Input: part model. Units: mm. Frame: model coordinates. Face numbers are marked on the shaded views. A direction names the side the tool comes from. Coordinates: 2 decimals unless noted, no trailing zeros. Order: outer loops, then holes, each group sorted by start corner. A loop starts at its lowest first (then second) coordinate and runs counter-clockwise, first axis right, second up. Notation, with made-up numbers: (65.5, 20) - (106.5, 20) arc R8 cw to (106.5, 33) - close; hole circle Ø5 at (57, -38.5). An arc over 180 degrees is marked (long way). Answer as CSV lines item,"result". Start each with the question number.
Item 1: Material intervals for line 1 along X through (y, z) = (37.5, 5.5); line 2 along Y through (x, z) = (1, 9.5); line 3 along Z through (x, y) = (-7, 48), sorted ascending.
Item 2: Section A-A (y = 69.5). Output: boundary loops of the cut face in (x, z), and give its area (3 significant figures).
Item 3: Section C-C (z = 12.75). Output: boundary loops of the cut face in (x, y).
Item 4: Access query for the marked faces 5, 6, 7, 8 and 9. Directions: +Z, -Z, +X, -X, +Y, -Y. A direction counts if a zero-diameter tool reaches every point of the face in a straight line with its end or side. Return the directions, or none.
Item 5: Section B-B (x = 11). Output: boundary loops of the cut face in (y, z), and give its area (3 significant figures).
Item 6: First-contact query: pin 1 (3 mm diameter, centred on y = 63, z = 19.5, fed in from +X); pin 2 (0.7 mm diameter, centred on x = 8.5, z = 21.5, fed in from +Y); pin 3 (12 mm diameter, centred on x = -1.5, z = 12.5, fed in from -Y); pin 4 (8 mm diameter, centred on x = 23.5, z = 13.5, fed in from -Y). Flat tips, straight axial feed; report the tip coordinate or a pass-through.
Item 7: Draft query along Y for the marked faces 1, 2, 3 and 4. Return one class per face: +Y half, -Y half, draft (parallel to the pull), parting line (faces both ways), or undercut.
Item 8: Section D-D (x = 22.6). Output: boundary loops of the cut face in (y, z).
from build123d import *

# Parameters (mm, degrees)
EXTRUDE_1_DEPTH      = 30
SKETCH_2_W           = 20.2
SKETCH_2_H           = 50
EXTRUDE_1_2_DEPTH    = 20
SKETCH_3_W           = 20.2
SKETCH_3_H           = 11
CUT_EXTRUDE_1_DEPTH  = 20
CUT_EXTRUDE_2_REACH  = 60.432
SKETCH_4_W           = 11
SKETCH_4_H           = 20
SKETCH_5_W           = 20.2
SKETCH_5_H           = 4.5
EXTRUDE_2_DEPTH      = 25
CUT_EXTRUDE_4_REACH  = 80.275
CUT_EXTRUDE_5_REACH  = 82.278
SKETCH_9_R           = 1.6
SKETCH_10_W          = 20.2
SKETCH_10_H          = 20
EXTRUDE_3_DEPTH      = 3
CUT_EXTRUDE_6_REACH  = 55.965
SKETCH_12_W          = 20.2
SKETCH_12_H          = 30
EXTRUDE_4_DEPTH      = 2
SKETCH_13_W          = 20.2
SKETCH_13_H          = 30
EXTRUDE_5_DEPTH      = 2
CUT_EXTRUDE_START    = -20.2
SKETCH_15_W          = 15.2
SKETCH_15_H          = 20
CUT_EXTRUDE_7_DEPTH  = 20.2
SKETCH_16_W          = 4.4
SKETCH_16_H          = 30
SKETCH_16_W_2        = 5.4
EXTRUDE_6_DEPTH      = 20
CUT_EXTRUDE_8_REACH  = 88.983
SKETCH_17_R          = 1.6
CHAMFER_1_SIZE       = 2.5
CUT_EXTRUDE_9_REACH  = 89.122
SKETCH_18_W          = 46.30929367
SKETCH_18_H          = 3
SKETCH_20_W          = 20.2
SKETCH_20_H          = 20
EXTRUDE_7_DEPTH      = 2.1
SKETCH_21_W          = 20.2
SKETCH_21_H          = 20
EXTRUDE_8_DEPTH      = 2.1
SKETCH_22_W          = 46.206629154
SKETCH_22_H          = 1
CUT_EXTRUDE_10_DEPTH = 30
SKETCH_23_W          = 42.922328926
SKETCH_23_H          = 4
CUT_EXTRUDE_11_DEPTH = 30
CUT_EXTRUDE_12_REACH = 85.656
SKETCH_24_W          = 4
SKETCH_24_H          = 48
SKETCH_25_W          = 15.2
SKETCH_25_H          = 20
CUT_EXTRUDE_13_DEPTH = 20.2
SKETCH_26_W          = 20.2
SKETCH_26_H          = 20
EXTRUDE_9_DEPTH      = 1
CHAMFER_2_SIZE       = 2
FILLET_1_R           = 1
CUT_EXTRUDE_14_DEPTH = 1


with BuildPart() as part:
    # Sketch 1 → Extrude 1 (new body)
    with BuildSketch(Plane(origin=(0, 0, 0), x_dir=(1, 0, 0), z_dir=(0, 1, 0))):
        Polygon((-7.6, 15), (-7.6, 0), (7.6, 0), (7.6, 15), (10.1, 15), (10.1, -2.5), (-10.1, -2.5), (-10.1, 15), align=None)
    extrude(amount=EXTRUDE_1_DEPTH)

    # Sketch 2 → Extrude 1 2 (add)
    with BuildSketch(Plane.XY.offset(2.5)):
        with Locations((0, 25)):
            Rectangle(SKETCH_2_W, SKETCH_2_H)
    extrude(amount=EXTRUDE_1_2_DEPTH)

    # Sketch 3 → Cut-Extrude 1 (cut)
    with BuildSketch(Plane(origin=(0, 50, 0), x_dir=(1, 0, 0), z_dir=(0, 1, 0))):
        with Locations((0, -12.5)):
            Rectangle(SKETCH_3_W, SKETCH_3_H)
    extrude(amount=-CUT_EXTRUDE_1_DEPTH, mode=Mode.SUBTRACT)

    # Sketch 4 → Cut-Extrude 2 (cut, up to next)
    with BuildSketch(Plane(origin=(10.1, 0, 0), x_dir=(0, 0, -1), z_dir=(1, 0, 0)), mode=Mode.PRIVATE) as cut_extrude_2_sk1:
        with Locations((-12.5, 15)):
            Rectangle(SKETCH_4_W, SKETCH_4_H)
    cut_extrude_2_tool1 = extrude(cut_extrude_2_sk1.sketch, amount=-CUT_EXTRUDE_2_REACH, mode=Mode.PRIVATE) & part.part
    add(cut_extrude_2_tool1.solids().sort_by_distance((10.1, 15, 12.5))[0], mode=Mode.SUBTRACT)

    # Sketch 5 → Extrude 2 (add)
    with BuildSketch(Plane(origin=(0, 50, 0), x_dir=(1, 0, 0), z_dir=(0, 1, 0))):
        with Locations((0, -4.75)):
            Rectangle(SKETCH_5_W, SKETCH_5_H)
        with Locations((0, -20.25)):
            Rectangle(SKETCH_5_W, SKETCH_5_H)
    extrude(amount=EXTRUDE_2_DEPTH)

    # Sketch 7 → Hole Wizard M3.5 _1 (revolve, cut)
    with BuildSketch(Plane(origin=(-5.1, 37.5, 2.5), x_dir=(0, 1, 0), z_dir=(1, 0, 0))):
        Polygon((0, 0), (0, 40.871247898), (1.45, 40), (1.45, 0), align=None)
    hole_wizard_m3_5_1 = revolve(axis=Axis((-5.1, 37.5, -3.85), (0, 0, 1)), mode=Mode.SUBTRACT)

    # Cut-Extrude 4: up to this face of the body (flat: up to its plane)
    cut_extrude_4_end = Plane(part.part.faces().sort_by_distance((0.022332689, 37.5, 22.5))[0])
    # Sketch 8 → Cut-Extrude 4 (cut, up to the picked face)
    with BuildSketch(Plane(origin=(0, 0, 2.5), x_dir=(-1, 0, 0), z_dir=(0, 0, -1)), mode=Mode.PRIVATE) as cut_extrude_4_sk1:
        with BuildLine():
            Line((3.5, 60.5), (3.5, 64.5))
            ThreePointArc((3.5, 64.5), (5.1, 66.1), (6.7, 64.5))
            Line((6.7, 64.5), (6.7, 60.5))
            ThreePointArc((6.7, 60.5), (5.1, 58.9), (3.5, 60.5))
        make_face()
    cut_extrude_4_tool1 = split(extrude(cut_extrude_4_sk1.sketch, amount=-CUT_EXTRUDE_4_REACH, mode=Mode.PRIVATE), bisect_by=cut_extrude_4_end, keep=Keep.BOTH, mode=Mode.PRIVATE)
    cut_extrude_4 = cut_extrude_4_tool1.solids().sort_by(Axis((-5.1, 62.5, 2.5), (0, 0, 1)))[0]
    add(cut_extrude_4, mode=Mode.SUBTRACT)

    # Sketch 9 → Cut-Extrude 5 (cut, up to next)
    with BuildSketch(Plane(origin=(-7.6, 0, 0), x_dir=(0, 0, -1), z_dir=(1, 0, 0)), mode=Mode.PRIVATE) as cut_extrude_5_sk1:
        with Locations((7.5, 25)):
            Circle(SKETCH_9_R)
    cut_extrude_5_tool1 = extrude(cut_extrude_5_sk1.sketch, amount=-CUT_EXTRUDE_5_REACH, mode=Mode.PRIVATE) & part.part
    # Sketch 9 → Cut-Extrude 5 (cut, up to next)
    with BuildSketch(Plane(origin=(-7.6, 0, 0), x_dir=(0, 0, -1), z_dir=(1, 0, 0)), mode=Mode.PRIVATE) as cut_extrude_5_sk2:
        with Locations((7.5, 5)):
            Circle(SKETCH_9_R)
    cut_extrude_5_tool2 = extrude(cut_extrude_5_sk2.sketch, amount=-CUT_EXTRUDE_5_REACH, mode=Mode.PRIVATE) & part.part
    cut_extrude_5_1 = cut_extrude_5_tool1.solids().sort_by_distance((-7.6, 25, -7.5))[0]
    add(cut_extrude_5_1, mode=Mode.SUBTRACT)
    cut_extrude_5_2 = cut_extrude_5_tool2.solids().sort_by_distance((-7.6, 5, -7.5))[0]
    add(cut_extrude_5_2, mode=Mode.SUBTRACT)
    cut_extrude_5 = cut_extrude_5_1 + cut_extrude_5_2  # Cut-Extrude 5 as one shape, for the pattern or mirror that repeats it

    # Mirror 1: Hole Wizard M3.5 _1, Cut-Extrude 4, Cut-Extrude 5 across plane
    add(hole_wizard_m3_5_1.mirror(Plane(origin=(0, 0, 0), x_dir=(0, 0, 1), z_dir=(1, 0, 0))), mode=Mode.SUBTRACT)
    add(cut_extrude_4.mirror(Plane(origin=(0, 0, 0), x_dir=(0, 0, 1), z_dir=(1, 0, 0))), mode=Mode.SUBTRACT)
    add(cut_extrude_5.mirror(Plane(origin=(0, 0, 0), x_dir=(0, 0, 1), z_dir=(1, 0, 0))), mode=Mode.SUBTRACT)

    # Sketch 10 → Extrude 3 (add)
    with BuildSketch(Plane(origin=(0, 75, 0), x_dir=(1, 0, 0), z_dir=(0, 1, 0))):
        with Locations((0, -12.5)):
            Rectangle(SKETCH_10_W, SKETCH_10_H)
    extrude(amount=EXTRUDE_3_DEPTH)

    # Sketch 11 → Cut-Extrude 6 (cut, up to next)
    with BuildSketch(Plane(origin=(0, 30, 0), x_dir=(1, 0, 0), z_dir=(0, 1, 0)), mode=Mode.PRIVATE) as cut_extrude_6_sk1:
        Polygon((10.1, -2.5), (10.1, 15), (7.6, 15), (7.6, 0), (-7.6, 0), (-7.6, 15), (-10.1, 15), (-10.1, -2.5), align=None)
    cut_extrude_6_tool1 = extrude(cut_extrude_6_sk1.sketch, amount=-CUT_EXTRUDE_6_REACH, mode=Mode.PRIVATE) & part.part
    add(cut_extrude_6_tool1.solids().sort_by_distance((9.832738, 30, -6.25))[0], mode=Mode.SUBTRACT)

    # Sketch 12 → Extrude 4 (add)
    with BuildSketch(Plane.XY.offset(22.5)):
        with Locations((0, 15)):
            Rectangle(SKETCH_12_W, SKETCH_12_H)
    extrude(amount=EXTRUDE_4_DEPTH)

    # Sketch 13 → Extrude 5 (add)
    with BuildSketch(Plane(origin=(0, 0, 2.5), x_dir=(-1, 0, 0), z_dir=(0, 0, -1))):
        with Locations((0, 15)):
            Rectangle(SKETCH_13_W, SKETCH_13_H)
    extrude(amount=EXTRUDE_5_DEPTH)

    # Sketch 15 → Cut-Extrude 7 (cut)
    with BuildSketch(Plane(origin=(10.1, 0, 0), x_dir=(0, 0, -1), z_dir=(1, 0, 0)).offset(CUT_EXTRUDE_START)):
        with Locations((-12.5, 15)):
            Rectangle(SKETCH_15_W, SKETCH_15_H)
    extrude(amount=CUT_EXTRUDE_7_DEPTH, mode=Mode.SUBTRACT)

    # Sketch 16 → Extrude 6 (add)
    with BuildSketch(Plane(origin=(10.1, 0, 0), x_dir=(0, 0, -1), z_dir=(1, 0, 0))):
        with Locations((-22.3, 15)):
            Rectangle(SKETCH_16_W, SKETCH_16_H)
        with Locations((-3.2, 15)):
            Rectangle(SKETCH_16_W_2, SKETCH_16_H)
    extrude(amount=EXTRUDE_6_DEPTH)

    # Cut-Extrude 8: up to this face of the body (flat: up to its plane)
    cut_extrude_8_end = Plane(part.part.faces().sort_by_distance((10, 15, 0.5))[0])
    # Sketch 17 → Cut-Extrude 8 (cut, up to the picked face)
    with BuildSketch(Plane.XY.offset(24.5), mode=Mode.PRIVATE) as cut_extrude_8_sk1:
        with Locations((22.6, 25)):
            Circle(SKETCH_17_R)
    cut_extrude_8_tool1 = split(extrude(cut_extrude_8_sk1.sketch, amount=-CUT_EXTRUDE_8_REACH, mode=Mode.PRIVATE), bisect_by=cut_extrude_8_end, keep=Keep.BOTH, mode=Mode.PRIVATE)
    # Sketch 17 → Cut-Extrude 8 (cut, up to the picked face)
    with BuildSketch(Plane.XY.offset(24.5), mode=Mode.PRIVATE) as cut_extrude_8_sk2:
        with Locations((22.6, 5)):
            Circle(SKETCH_17_R)
    cut_extrude_8_tool2 = split(extrude(cut_extrude_8_sk2.sketch, amount=-CUT_EXTRUDE_8_REACH, mode=Mode.PRIVATE), bisect_by=cut_extrude_8_end, keep=Keep.BOTH, mode=Mode.PRIVATE)
    add(cut_extrude_8_tool1.solids().sort_by(Axis((22.6, 25, 24.5), (0, 0, -1)))[0], mode=Mode.SUBTRACT)
    add(cut_extrude_8_tool2.solids().sort_by(Axis((22.6, 5, 24.5), (0, 0, -1)))[0], mode=Mode.SUBTRACT)

    # Chamfer 1
    chamfer_1_edges = [part.edges().sort_by_distance(p)[0] for p in [
        (30.1, 0, 22.3),
        (30.1, 0, 3.2),
        (30.1, 30, 3.2),
        (30.1, 30, 22.3),
    ]]
    chamfer(chamfer_1_edges, length=CHAMFER_1_SIZE)

    # Cut-Extrude 9: up to this face of the body (flat: up to its plane)
    cut_extrude_9_end = Plane(part.part.faces().sort_by_distance((0, 78, 12.5))[0])
    # Sketch 18 → Cut-Extrude 9 (cut, up to the picked face)
    with BuildSketch(Plane.XZ, mode=Mode.PRIVATE) as cut_extrude_9_sk1:
        with Locations((8.75, 0.5)):
            Rectangle(SKETCH_18_W, SKETCH_18_H)
    cut_extrude_9_tool1 = split(extrude(cut_extrude_9_sk1.sketch, amount=-CUT_EXTRUDE_9_REACH, mode=Mode.PRIVATE), bisect_by=cut_extrude_9_end, keep=Keep.BOTH, mode=Mode.PRIVATE)
    add(cut_extrude_9_tool1.solids().sort_by(Axis((8.75, 0, 0.5), (0, 1, 0)))[0], mode=Mode.SUBTRACT)

    # Sketch 20 → Extrude 7 (add)
    with BuildSketch(Plane.XY.offset(4.9)):
        with Locations((0, 15)):
            Rectangle(SKETCH_20_W, SKETCH_20_H)
    extrude(amount=EXTRUDE_7_DEPTH)

    # Sketch 21 → Extrude 8 (add)
    with BuildSketch(Plane(origin=(0, 0, 20.1), x_dir=(-1, 0, 0), z_dir=(0, 0, -1))):
        with Locations((0, 15)):
            Rectangle(SKETCH_21_W, SKETCH_21_H)
    extrude(amount=EXTRUDE_8_DEPTH)

    # Sketch 22 → Cut-Extrude 10 (cut)
    with BuildSketch(Plane(origin=(0, 30, 0), x_dir=(1, 0, 0), z_dir=(0, 1, 0))):
        with Locations((8.75, -2)):
            Rectangle(SKETCH_22_W, SKETCH_22_H)
    extrude(amount=-CUT_EXTRUDE_10_DEPTH, mode=Mode.SUBTRACT)

    # Sketch 23 → Cut-Extrude 11 (cut)
    with BuildSketch(Plane(origin=(0, 30, 0), x_dir=(1, 0, 0), z_dir=(0, 1, 0))):
        with Locations((8.75, -24.5)):
            Rectangle(SKETCH_23_W, SKETCH_23_H)
    extrude(amount=-CUT_EXTRUDE_11_DEPTH, mode=Mode.SUBTRACT)

    # Sketch 24 → Cut-Extrude 12 (cut, up to next)
    with BuildSketch(Plane(origin=(10.1, 0, 0), x_dir=(0, 0, -1), z_dir=(1, 0, 0)), mode=Mode.PRIVATE) as cut_extrude_12_sk1:
        with Locations((-22.5, 54)):
            Rectangle(SKETCH_24_W, SKETCH_24_H)
    cut_extrude_12_tool1 = extrude(cut_extrude_12_sk1.sketch, amount=-CUT_EXTRUDE_12_REACH, mode=Mode.PRIVATE) & part.part
    # Sketch 24 → Cut-Extrude 12 (cut, up to next)
    with BuildSketch(Plane(origin=(10.1, 0, 0), x_dir=(0, 0, -1), z_dir=(1, 0, 0)), mode=Mode.PRIVATE) as cut_extrude_12_sk2:
        with Locations((-2.5, 54)):
            Rectangle(SKETCH_24_W, SKETCH_24_H)
    cut_extrude_12_tool2 = extrude(cut_extrude_12_sk2.sketch, amount=-CUT_EXTRUDE_12_REACH, mode=Mode.PRIVATE) & part.part
    add(cut_extrude_12_tool1.solids().sort_by_distance((10.1, 54, 22.5))[0], mode=Mode.SUBTRACT)
    add(cut_extrude_12_tool2.solids().sort_by_distance((10.1, 54, 2.5))[0], mode=Mode.SUBTRACT)

    # Sketch 25 → Cut-Extrude 13 (cut)
    with BuildSketch(Plane(origin=(10.1, 0, 0), x_dir=(0, 0, -1), z_dir=(1, 0, 0)).offset(CUT_EXTRUDE_START)):
        with Locations((-12.5, 15)):
            Rectangle(SKETCH_25_W, SKETCH_25_H)
    extrude(amount=CUT_EXTRUDE_13_DEPTH, mode=Mode.SUBTRACT)

    # Sketch 26 → Extrude 9 (add)
    with BuildSketch(Plane.XY.offset(4.9)):
        with Locations((0, 15)):
            Rectangle(SKETCH_26_W, SKETCH_26_H)
    extrude(amount=EXTRUDE_9_DEPTH)

    # Chamfer 2
    chamfer_2_edges = [part.edges().sort_by_distance(p)[0] for p in [
        (0, 30, 4.5),
        (0, 30, 20.5),
    ]]
    chamfer(chamfer_2_edges, length=CHAMFER_2_SIZE - 0.0001)  # a hair under: the kernel refuses the full size

    # Fillet 1
    fillet_1_edges = [part.edges().sort_by_distance(p)[0] for p in [
        (0, 78, 20.5),
        (0, 78, 4.5),
    ]]
    fillet(fillet_1_edges, radius=FILLET_1_R)

    # Sketch 27 → Cut-Extrude 14 (cut)
    with BuildSketch(Plane.XY.offset(5.9)):
        Polygon((10.1, 0), (27.6, 0), (30.1, 2.5), (30.1, 27.5), (27.6, 30), (10.1, 30), (10.1, 25), (-10.1, 25), (-10.1, 5), (10.1, 5), align=None)
    extrude(amount=-CUT_EXTRUDE_14_DEPTH, mode=Mode.SUBTRACT)


solid = part.part
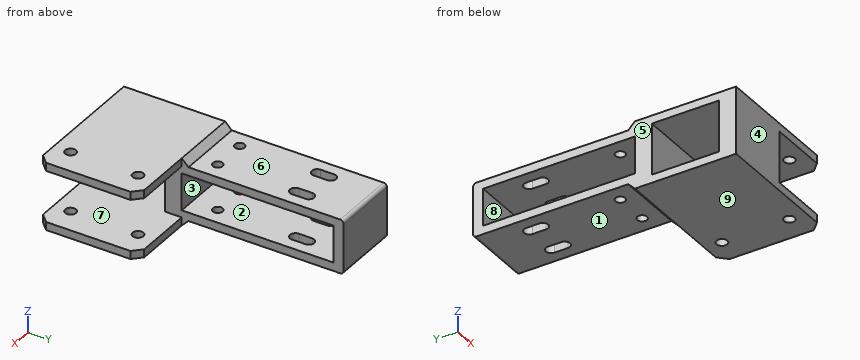
Determined:
1,line 1,"x = -10.1 to -6.55, -3.65 to 3.65, 6.55 to 10.1"
1,line 2,"y = 0 to 5, 25 to 30, 75 to 78"
1,line 3,"z = 4.5 to 7, 18 to 20.5"
2,outline,"(-10.1, 4.5) - (10.1, 4.5) - (10.1, 7) - (-10.1, 7) - close; (-10.1, 18) - (10.1, 18) - (10.1, 20.5) - (-10.1, 20.5) - close"
2,area,"101 mm^2"
3,outline,"(-10.1, 0) - (10.1, 0) - (10.1, 5) - (-10.1, 5) - close; (-10.1, 25) - (10.1, 25) - (10.1, 30) - (-10.1, 30) - close; (-10.1, 75) - (10.1, 75) - (10.1, 78) - (-10.1, 78) - close"
4,face 5,"+Z, -Z, -X, +Y, -Y"
4,face 6,"+Z, +X, -X, +Y"
4,face 7,"+X"
4,face 8,"+X, -X"
4,face 9,"-Z, +X, -X, +Y, -Y"
5,outline,"(0, 2.5) - (30, 2.5) - (30, 4.9) - (0, 4.9) - close; (0, 20.1) - (30, 20.1) - (30, 22.5) - (0, 22.5) - close"
5,area,"144 mm^2"
6,pin 1,"stops at x = 10.1"
6,pin 2,"stops at y = 31.35"
6,pin 3,"stops at y = 0"
6,pin 4,"passes through"
7,face 1,"draft"
7,face 2,"undercut"
7,face 3,"undercut"
7,face 4,"-Y half"
8,outline,"(0, 2.5) - (3.4, 2.5) - (3.4, 4.9) - (0, 4.9) - close; (0, 20.1) - (3.4, 20.1) - (3.4, 22.5) - (0, 22.5) - close; (6.6, 2.5) - (23.4, 2.5) - (23.4, 4.9) - (6.6, 4.9) - close; (6.6, 20.1) - (23.4, 20.1) - (23.4, 22.5) - (6.6, 22.5) - close; (26.6, 2.5) - (30, 2.5) - (30, 4.9) - (26.6, 4.9) - close; (26.6, 20.1) - (30, 20.1) - (30, 22.5) - (26.6, 22.5) - close"
